```python
from build123d import *

# Parameters (mm, degrees)
BOSS_EXTRUDE1_DEPTH = 4
BOSS_EXTRUDE2_START = -4
BOSS_EXTRUDE2_DEPTH = 37
SKETCH3_R           = 4
SKETCH3_R_2         = 2.5
CUT_EXTRUDE1_DEPTH  = 109.592312231
SKETCH4_W           = 73.911051306
SKETCH4_H           = 52.5
BOSS_EXTRUDE3_DEPTH = 4
SKETCH5_R           = 1.9
CUT_EXTRUDE2_DEPTH  = 37
BOSS_EXTRUDE4_START = -4
BOSS_EXTRUDE4_DEPTH = 37
SKETCH7_R           = 1.9
SKETCH7_R_2         = 7.5
CUT_EXTRUDE4_DEPTH  = 4
SKETCH8_W           = 80
SKETCH8_H           = 70
SKETCH8_R           = 1.75
BOSS_EXTRUDE5_DEPTH = 4


with BuildPart() as part:
    # Sketch1 → Boss-Extrude1 (new body)
    with BuildSketch(Plane(origin=(0, 0, 0), x_dir=(1, 0, 0), z_dir=(0, 1, 0))):
        Polygon((40.955525653, 11.5), (59.955525653, 11.5), (59.955525653, 15.5), (-59.955525653, 15.5), (-59.955525653, 11.5), (-40.955525653, 11.5), (-40.955525653, -11.5), (-59.955525653, -11.5), (-59.955525653, -15.5), (59.955525653, -15.5), (59.955525653, -11.5), (40.955525653, -11.5), align=None)
    extrude(amount=BOSS_EXTRUDE1_DEPTH)

    # Sketch2 → Boss-Extrude2 (add)
    with BuildSketch(Plane(origin=(0, 4, 0), x_dir=(1, 0, 0), z_dir=(0, 1, 0)).offset(BOSS_EXTRUDE2_START)):
        Polygon((-36.955525653, 15.5), (-59.955525653, 15.5), (-59.955525653, 11.5), (-40.955525653, 11.5), (-40.955525653, -11.5), (-59.955525653, -11.5), (-59.955525653, -15.5), (-36.955525653, -15.5), align=None)
        Polygon((36.955525653, -15.5), (36.955525653, 15.5), (59.955525653, 15.5), (59.955525653, 11.5), (40.955525653, 11.5), (40.955525653, -11.5), (59.955525653, -11.5), (59.955525653, -15.5), align=None)
    extrude(amount=BOSS_EXTRUDE2_DEPTH)

    # Sketch3 → Cut-Extrude1 (cut, through all)
    with BuildSketch(Plane.ZY.offset(40.955525653)):
        with Locations((0, 15.5)):
            Circle(SKETCH3_R)
        with Locations((0, 24.5)):
            Circle(SKETCH3_R_2)
    extrude(amount=-CUT_EXTRUDE1_DEPTH, mode=Mode.SUBTRACT)

    # Sketch4 → Boss-Extrude3 (add)
    with BuildSketch(Plane(origin=(0, 4, 0), x_dir=(1, 0, 0), z_dir=(0, 1, 0))):
        with Locations((0, 8.75)):
            Rectangle(SKETCH4_W, SKETCH4_H)
    extrude(amount=-BOSS_EXTRUDE3_DEPTH)

    # Sketch5 → Cut-Extrude2 (cut)
    with BuildSketch(Plane(origin=(0, 4, 0), x_dir=(1, 0, 0), z_dir=(0, 1, 0))):
        with Locations(Location((-18.35, 30.080617362, 0), (0, 0, 270))):
            Circle(SKETCH5_R)
        with Locations(Location((18.35, 30.080617362, 0), (0, 0, 270))):
            Circle(SKETCH5_R)
        with Locations(Location((18.35, -13.219382638, 0), (0, 0, 270))):
            Circle(SKETCH5_R)
        with Locations(Location((-18.35, -13.219382638, 0), (0, 0, 270))):
            Circle(SKETCH5_R)
    extrude(amount=-CUT_EXTRUDE2_DEPTH, mode=Mode.SUBTRACT)

    # Sketch6 → Boss-Extrude4 (add)
    with BuildSketch(Plane(origin=(0, 4, 0), x_dir=(1, 0, 0), z_dir=(0, 1, 0)).offset(BOSS_EXTRUDE4_START)):
        Polygon((-36.955525653, 15.5), (-36.955525653, 35), (36.955525653, 35), (36.955525653, 15.5), (40.955525653, 15.5), (40.955525653, 35), (51, 35), (51, 39), (-51, 39), (-51, 35), (-40.955525653, 35), (-40.955525653, 15.5), align=None)
    extrude(amount=BOSS_EXTRUDE4_DEPTH)

    # Sketch7 → Cut-Extrude4 (cut)
    with BuildSketch(Plane(origin=(0, 0, -39), x_dir=(-1, 0, 0), z_dir=(0, 0, -1))):
        with Locations((-47.5, 30)):
            Circle(SKETCH7_R)
        with Locations((47.5, 30)):
            Circle(SKETCH7_R)
        with Locations((47.5, 5)):
            Circle(SKETCH7_R)
        with Locations((-47.5, 5)):
            Circle(SKETCH7_R)
        with Locations((0, 17.5)):
            Circle(SKETCH7_R_2)
    extrude(amount=-CUT_EXTRUDE4_DEPTH, mode=Mode.SUBTRACT)

    # Sketch8 → Boss-Extrude5 (add)
    with BuildSketch(Plane(origin=(0, 0, -39), x_dir=(-1, 0, 0), z_dir=(0, 0, -1))):
        with Locations((0, 72)):
            Rectangle(SKETCH8_W, SKETCH8_H)
        with Locations((-32, 90.5)):
            Circle(SKETCH8_R, mode=Mode.SUBTRACT)
        with Locations((-32, 62.5)):
            Circle(SKETCH8_R, mode=Mode.SUBTRACT)
        with Locations((16.5, 47)):
            Circle(SKETCH8_R, mode=Mode.SUBTRACT)
    extrude(amount=-BOSS_EXTRUDE5_DEPTH)


solid = part.part
```
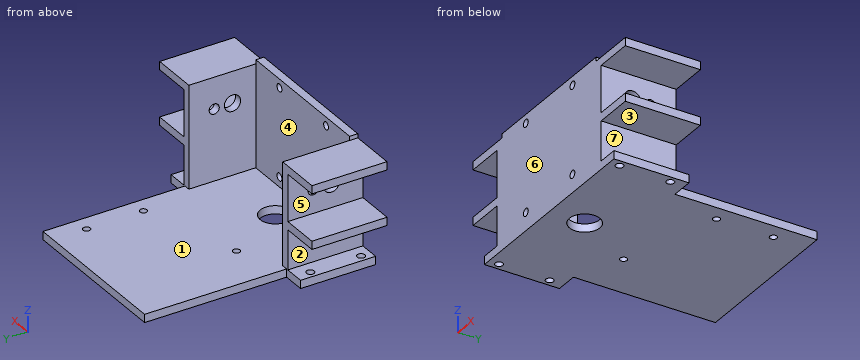
Source: CAD feature listing. Evaluate the final solid. Frame: model axes, mm. Face numbers are marked on the shaded views. A direction names the side the tool comes from. Coordinates: 2 decimals unless noted, no trailing zeros. Order: outer loops, then holes, each group sorted by start corner. A loop starts at its lowest first (then second) coordinate and runs counter-clockwise, first axis right, second up. Notation, with made-up numbers: (-7.5, 50) - (39.5, 50) arc R32 cw to (39.5, 87) - close; hole circle Ø7 at (65, 39). An arc over 180 degrees is marked (long way). One line per item, written item: value.
1) Cut plane C-C on z = -22.5. Output: boundary loops of the cut face in (x, y).
Computed values:
outline: (-40.96, 0) - (40.96, 0) - (40.96, 37) - (36.96, 37) - (36.96, 4) - (-36.96, 4) - (-36.96, 37) - (-40.96, 37) - close
2) Mould query, pull axis X, two halves, no side actions, for the marked faces 1, 2 and 3. Classes: released by +X, released by -X, zero draft, split by the parting line, or undercut.
Computed values:
face 1: undercut
face 2: released by -X
face 3: zero draft
3) Cut plane A-A on x = -43. Output: boundary loops of the cut face in (y, z), plus the area to 3 significant figures.
Computed values:
outline: (0, -39) - (37, -39) - (37, -35) - (0, -35) - close; (0, -15.5) - (37, -15.5) - (37, -11.5) - (0, -11.5) - close; (0, 11.5) - (37, 11.5) - (37, 15.5) - (0, 15.5) - close
area: 444 mm^2
4) Cut plane B-B on y = 30. State how many separate pieces and enclosed holes the cut face has, plus the area to 3 significant figures.
Computed values:
separate pieces: 3
enclosed holes: 0
area: 1,090 mm^2
5) Reachability of the marked faces 4, 5, 6 and 7 from +Z, -Z, +X, -X, +Y, -Y: full face, straight path, thin tool, end or side. Return the list, or none.
Computed values:
face 4: +Z, +Y
face 5: -X, +Y, -Y
face 6: +Z, -Z, +X, -X, -Y
face 7: +X, +Y, -Y
6) Cut plane D-D on y = 47. Output: boundary loops of the cut face in (x, z).
Computed values:
outline: (-40, -39) - (-18.25, -39) - (-18.25, -35) - (-40, -35) - close; (-14.75, -39) - (40, -39) - (40, -35) - (-14.75, -35) - close
7) Ray query, line 1 (Y direction, x = 47.5, z = -35.9); line 2 (Y direction, x = -37.85, z = 0); line 3 (Z direction, x = 18, y = 3). Return the intervals inside material, ascending. Write a range as [from, to].
Computed values:
line 1: y = [0, 3.1], [6.9, 28.1], [31.9, 37]
line 2: y = [0, 11.5], [19.5, 22], [27, 37]
line 3: z = [-39, -31.95], [-28.21, 11.35], [15.09, 17.5]
8) Contact query for flat-ended pins moving along their axis: pin 1 (7 mm diameter, centred on x = 53.5, y = 24.5, fed in from +Z); pin 2 (2 mm diameter, centred on x = 23, z = -11.5, fed in from +Y); pin 3 (7 mm diameter, centred on x = -50.5, z = -12.5, fed in from +Y); pin 4 (4 mm diameter, centred on x = -42.5, y = 74.5, fed in from -Z). Output: stop coordinate, or through.
Computed values:
pin 1: stops at z = 15.5
pin 2: stops at y = 4
pin 3: stops at y = 37
pin 4: passes through
